Part model, mm, in its own coordinate system. Give positions to 0.01 mm unless a question says otherwise; leave off trailing zeros. Order: outer loops, then holes, each group sorted by start corner. A loop starts at its lowest first (then second) coordinate and runs counter-clockwise, first axis right, second up. Notation, with made-up numbers: M 11,-10.75 L 39,-10.75 A17 ccw 39,5.25 Z; hole C 57,-15 d9. An arc over 180 degrees is marked long. Write each question's results on one line, items separated by ' | '. Start each with the question number.
from build123d import *

# Parameters (mm, degrees)
BOSS_EXTRUDE1_DEPTH = 1.5
SKETCH6_R           = 1
CUT_EXTRUDE1_DEPTH  = 10
FILLET4_R           = 1.5
FILLET5_R           = 3


# Read off the part's stored shape, not the designer's step: AdvancedHole1
with BuildPart() as part:
    # Sketch1 → Boss-Extrude1 (new body)
    with BuildSketch(Plane.XY):
        Polygon((-132.514999879, 63.173696093), (13.284995002, 63.173696093), (13.284995002, -23.784888353), (18.416457767, -33.534813854), (46.668669763, -49.846236055), (26.202746282, -85.294255348), (6.148371034, -73.7158564), (-19.700470814, -64.307647377), (-16.953396025, -56.760121426), (-32.457645619, -54.026303907), (-132.514999879, -54.026303907), align=None)
    extrude(amount=BOSS_EXTRUDE1_DEPTH)

    # Sketch6 → Cut-Extrude1 (cut)
    with BuildSketch(Plane(origin=(0, 0, 0), x_dir=(-1, 0, 0), z_dir=(0, 0, -1))):
        with Locations((125.729523879, 52.403696093)):
            Circle(SKETCH6_R)
        with Locations((106.929523879, -34.896303907)):
            Circle(SKETCH6_R)
        with Locations((30.929523879, -17.596303907)):
            Circle(SKETCH6_R)
        with Locations((31.129523879, 19.803696093)):
            Circle(SKETCH6_R)
        with Locations((-7.470476121, 40.003696093)):
            Circle(SKETCH6_R)
        with Locations((1.029523879, -34.496303907)):
            Circle(SKETCH6_R)
        with Locations((10.929523879, -60.496303907)):
            Circle(SKETCH6_R)
        with Locations((-37.470476121, -52.796303907)):
            Circle(SKETCH6_R)
        with Locations((-24.070476121, -75.996303907)):
            Circle(SKETCH6_R)
        with Locations((107.229523879, 19.603696093)):
            Circle(SKETCH6_R)
    extrude(amount=-CUT_EXTRUDE1_DEPTH, mode=Mode.SUBTRACT)

    # AdvancedHole1 outline → AdvancedHole1 (revolve, cut)
    with BuildSketch(Plane(origin=(37.470476121, -52.796303907, 0), x_dir=(1, 0, 0), z_dir=(0, -1, 0))):
        Polygon((2.2, 0), (1, 1.2), (1, 0), align=None)
    revolve(axis=Axis((37.470476121, -52.796303907, 0), (0, 0, 1)), mode=Mode.SUBTRACT)

    # AdvancedHole1 2 outline → AdvancedHole1 2 (revolve, cut)
    with BuildSketch(Plane(origin=(24.070476121, -75.996303907, 0), x_dir=(1, 0, 0), z_dir=(0, -1, 0))):
        Polygon((2.2, 0), (1, 1.2), (1, 0), align=None)
    revolve(axis=Axis((24.070476121, -75.996303907, 0), (0, 0, 1)), mode=Mode.SUBTRACT)

    # AdvancedHole1 3 outline → AdvancedHole1 3 (revolve, cut)
    with BuildSketch(Plane(origin=(-10.929523879, -60.496303907, 0), x_dir=(1, 0, 0), z_dir=(0, -1, 0))):
        Polygon((2.2, 0), (1, 1.2), (1, 0), align=None)
    revolve(axis=Axis((-10.929523879, -60.496303907, 0), (0, 0, 1)), mode=Mode.SUBTRACT)

    # AdvancedHole1 4 outline → AdvancedHole1 4 (revolve, cut)
    with BuildSketch(Plane(origin=(-1.029523879, -34.496303907, 0), x_dir=(1, 0, 0), z_dir=(0, -1, 0))):
        Polygon((2.2, 0), (1, 1.2), (1, 0), align=None)
    revolve(axis=Axis((-1.029523879, -34.496303907, 0), (0, 0, 1)), mode=Mode.SUBTRACT)

    # AdvancedHole1 5 outline → AdvancedHole1 5 (revolve, cut)
    with BuildSketch(Plane(origin=(-30.929523879, -17.596303907, 0), x_dir=(1, 0, 0), z_dir=(0, -1, 0))):
        Polygon((2.2, 0), (1, 1.2), (1, 0), align=None)
    revolve(axis=Axis((-30.929523879, -17.596303907, 0), (0, 0, 1)), mode=Mode.SUBTRACT)

    # AdvancedHole1 6 outline → AdvancedHole1 6 (revolve, cut)
    with BuildSketch(Plane(origin=(-106.929523879, -34.896303907, 0), x_dir=(1, 0, 0), z_dir=(0, -1, 0))):
        Polygon((2.2, 0), (1, 1.2), (1, 0), align=None)
    revolve(axis=Axis((-106.929523879, -34.896303907, 0), (0, 0, 1)), mode=Mode.SUBTRACT)

    # AdvancedHole1 7 outline → AdvancedHole1 7 (revolve, cut)
    with BuildSketch(Plane(origin=(-125.729523879, 52.403696093, 0), x_dir=(1, 0, 0), z_dir=(0, -1, 0))):
        Polygon((2.2, 0), (1, 1.2), (1, 0), align=None)
    revolve(axis=Axis((-125.729523879, 52.403696093, 0), (0, 0, 1)), mode=Mode.SUBTRACT)

    # AdvancedHole1 8 outline → AdvancedHole1 8 (revolve, cut)
    with BuildSketch(Plane(origin=(-31.129523879, 19.803696093, 0), x_dir=(1, 0, 0), z_dir=(0, -1, 0))):
        Polygon((2.2, 0), (1, 1.2), (1, 0), align=None)
    revolve(axis=Axis((-31.129523879, 19.803696093, 0), (0, 0, 1)), mode=Mode.SUBTRACT)

    # AdvancedHole1 9 outline → AdvancedHole1 9 (revolve, cut)
    with BuildSketch(Plane(origin=(-107.229523879, 19.603696093, 0), x_dir=(1, 0, 0), z_dir=(0, -1, 0))):
        Polygon((2.2, 0), (1, 1.2), (1, 0), align=None)
    revolve(axis=Axis((-107.229523879, 19.603696093, 0), (0, 0, 1)), mode=Mode.SUBTRACT)

    # AdvancedHole1 10 outline → AdvancedHole1 10 (revolve, cut)
    with BuildSketch(Plane(origin=(7.470476121, 40.003696093, 0), x_dir=(1, 0, 0), z_dir=(0, -1, 0))):
        Polygon((2.2, 0), (1, 1.2), (1, 0), align=None)
    revolve(axis=Axis((7.470476121, 40.003696093, 0), (0, 0, 1)), mode=Mode.SUBTRACT)

    # Fillet4
    fillet4_edges = [part.edges().sort_by_distance(p)[0] for p in [
        (-132.514999879, 63.173696093, 0.75),
        (13.284995002, 63.173696093, 0.75),
        (46.668669763, -49.846236055, 0.75),
        (26.202746282, -85.294255348, 0.75),
        (-132.514999879, -54.026303907, 0.75),
    ]]
    fillet(fillet4_edges, radius=FILLET4_R)

    # Fillet5
    fillet5_edges = [part.edges().sort_by_distance(p)[0] for p in [
        (13.284995002, -23.784888353, 0.75),
        (18.416457767, -33.534813854, 0.75),
        (-19.700470814, -64.307647377, 0.75),
        (-16.953396025, -56.760121426, 0.75),
        (-32.457645619, -54.026303907, 0.75),
    ]]
    fillet(fillet5_edges, radius=FILLET5_R)


solid = part.part
(1) Saw through at C-C on y = 30. Give the cut face in (x, z) (3 decimals), plus the area to 3 significant figures.
(2) Saw through at A-A on z = 0.55. Give the number of separate pieces and of enclosed holes in the cut face, plus the area to 3 significant figures.
(3) Saw through at B-B on x = -36. Give the cut face in (y, z), plus the area to 3 significant figures.
(4) Probe L1, parallel to Y at x = -44.5, z = 0.3; L2, parallel to X at y = 7, z = 1.3 (3 decimals); L3, parallel to X at y = 41, z = 0.9 (3 decimals). List the from-to ranges inside material, lowest first.
Taken from the geometry:
1) outline: M -132.515,0 L 13.285,0 L 13.285,1.5 L -132.515,1.5 Z | area: 219 mm²
2) separate pieces: 1 | enclosed holes: 10 | area: 18,700 mm²
3) outline: M -54.03,0 L 63.17,0 L 63.17,1.5 L -54.03,1.5 Z | area: 176 mm²
4) L1: y = -54.03 to 63.17 | L2: x = -132.515 to 13.285 | L3: x = -132.515 to 6.635, 8.306 to 13.285
